```python
from build123d import *

# Parameters (mm, degrees)
SKETCH1_W            = 80
SKETCH1_H            = 50
BOSS_EXTRUDE1_DEPTH  = 90
SKETCH2_W            = 20
SKETCH2_H            = 30
CUT_EXTRUDE1_DEPTH   = 90
BOSS_EXTRUDE2_DEPTH  = 20
CUT_EXTRUDE2_DEPTH   = 127
BOSS_EXTRUDE10_DEPTH = 38
BOSS_EXTRUDE16_DEPTH = 38
BOSS_EXTRUDE17_DEPTH = 38
SKETCH13_W           = 30
SKETCH13_H           = 50
CUT_EXTRUDE4_DEPTH   = 38
SKETCH14_W           = 100
SKETCH14_H           = 90
CUT_EXTRUDE5_DEPTH   = 38
SKETCH15_W           = 106.776830175
SKETCH15_H           = 78.518203409
CUT_EXTRUDE6_DEPTH   = 38
BOSS_EXTRUDE18_DEPTH = 10
CUT_EXTRUDE7_DEPTH   = 10
BOSS_EXTRUDE19_DEPTH = 112
SKETCH19_W           = 80
SKETCH19_H           = 90
CUT_EXTRUDE8_DEPTH   = 112
SKETCH20_W           = 107.666200856
SKETCH20_H           = 176.074092784
CUT_EXTRUDE9_DEPTH   = 112
SKETCH21_W           = 20
SKETCH21_H           = 60
CUT_EXTRUDE10_DEPTH  = 112
SKETCH27_W           = 22.568644797
SKETCH27_H           = 9.839278278
BOSS_EXTRUDE22_DEPTH = 20
BOSS_EXTRUDE24_DEPTH = 91
SKETCH32_W           = 16.460176991
SKETCH32_H           = 60
CUT_EXTRUDE13_DEPTH  = 101
CUT_EXTRUDE14_DEPTH  = 101
BOSS_EXTRUDE25_DEPTH = 5
SKETCH35_W           = 20
SKETCH35_H           = 60
CUT_EXTRUDE15_DEPTH  = 152
BOSS_EXTRUDE27_DEPTH = 20
SKETCH42_W           = 25
SKETCH42_H           = 10
BOSS_EXTRUDE29_DEPTH = 20
BOSS_EXTRUDE30_DEPTH = 20
BOSS_EXTRUDE31_DEPTH = 20
SKETCH46_W           = 60
SKETCH46_H           = 50
CUT_EXTRUDE19_DEPTH  = 20
CUT_EXTRUDE20_DEPTH  = 20
CUT_EXTRUDE21_DEPTH  = 10


with BuildPart() as part:
    # Sketch1 → Boss-Extrude1 (new body)
    with BuildSketch(Plane(origin=(0, 0, 0), x_dir=(1, 0, 0), z_dir=(0, 1, 0))):
        with Locations((40, 25)):
            Rectangle(SKETCH1_W, SKETCH1_H)
    extrude(amount=BOSS_EXTRUDE1_DEPTH)

    # Sketch2 → Cut-Extrude1 (cut)
    with BuildSketch(Plane(origin=(0, 90, 0), x_dir=(1, 0, 0), z_dir=(0, 1, 0))):
        with Locations((10, 15)):
            Rectangle(SKETCH2_W, SKETCH2_H)
    extrude(amount=-CUT_EXTRUDE1_DEPTH, mode=Mode.SUBTRACT)

    # Sketch3 → Boss-Extrude2 (add)
    with BuildSketch(Plane(origin=(80, 0, 0), x_dir=(0, 0, -1), z_dir=(1, 0, 0))):
        Polygon((20, 0), (50, 0), (50, 40), (30, 40), align=None)
    extrude(amount=BOSS_EXTRUDE2_DEPTH)

    # Sketch4 → Cut-Extrude2 (cut)
    with BuildSketch(Plane(origin=(0, 90, 0), x_dir=(1, 0, 0), z_dir=(0, 1, 0))):
        Polygon((60, 0), (80, 20), (80, 0), align=None)
    extrude(amount=-CUT_EXTRUDE2_DEPTH, mode=Mode.SUBTRACT)

    # Sketch7 → Boss-Extrude10 (add)
    with BuildSketch(Plane(origin=(38.787878788, 9.696969697, 38.787878788), x_dir=(0.717740563, -0.168880132, -0.675520529), z_dir=(0.696310624, 0.174077656, 0.696310624))):
        Polygon((29.554023164, -4.850712501), (85.284466846, 4.850712501), (85.284466846, 46.081768757), align=None)
    extrude(amount=-BOSS_EXTRUDE10_DEPTH)

    # Sketch10 → Boss-Extrude16 (add)
    with BuildSketch(Plane(origin=(39.036144578, 8.674698795, 39.036144578), x_dir=(0.715575428, -0.15153362, -0.68190129), z_dir=(0.698535473, 0.155230105, 0.698535473))):
        Polygon((57.246034218, 92.195444573), (15.321732688, 85.687530838), (29.296499865, -4.338609156), (85.195568572, 4.338609156), (85.195568572, 46.23657111), align=None)
    extrude(amount=-BOSS_EXTRUDE16_DEPTH)

    # Sketch11 → Boss-Extrude17 (add)
    with BuildSketch(Plane(origin=(100, 0, 0), x_dir=(0, 0, -1), z_dir=(1, 0, 0))):
        Polygon((20, 0), (29.088944068, 40.900248307), (30, 40), align=None)
    extrude(amount=-BOSS_EXTRUDE17_DEPTH)

    # Sketch13 → Cut-Extrude4 (cut)
    with BuildSketch(Plane(origin=(80, 0, 0), x_dir=(0, 0, -1), z_dir=(1, 0, 0))):
        with Locations((35, 65)):
            Rectangle(SKETCH13_W, SKETCH13_H)
    extrude(amount=CUT_EXTRUDE4_DEPTH, mode=Mode.SUBTRACT)

    # Sketch14 → Cut-Extrude5 (cut)
    with BuildSketch(Plane(origin=(0, 0, -50), x_dir=(-1, 0, 0), z_dir=(0, 0, -1))):
        with Locations((-50, 45)):
            Rectangle(SKETCH14_W, SKETCH14_H)
    extrude(amount=CUT_EXTRUDE5_DEPTH, mode=Mode.SUBTRACT)

    # Sketch15 → Cut-Extrude6 (cut)
    with BuildSketch(Plane.XZ):
        with Locations((53.388415088, -10.740898295)):
            Rectangle(SKETCH15_W, SKETCH15_H)
    extrude(amount=CUT_EXTRUDE6_DEPTH, mode=Mode.SUBTRACT)

    # Sketch16 → Boss-Extrude18 (add)
    with BuildSketch(Plane(origin=(0, 0, 0), x_dir=(-1, 0, 0), z_dir=(0, -1, 0))):
        Polygon((-60, -20), (-60, -40), (-40, -70), (0, -70), (0, -30), (-20, -30), (-20, 0), (-40, 0), align=None)
    extrude(amount=-BOSS_EXTRUDE18_DEPTH)

    # Sketch17 → Cut-Extrude7 (cut)
    with BuildSketch(Plane(origin=(0, 39.026548673, 44.601769912), x_dir=(-1, 0, 0), z_dir=(0, -0.658504608, -0.752576695))):
        Polygon((-20, 67.731902524), (0, -38.569555604), (-40, -38.569555604), (-60, 67.731902524), align=None)
    extrude(amount=-CUT_EXTRUDE7_DEPTH, mode=Mode.SUBTRACT)

    # Sketch18 → Boss-Extrude19 (add)
    with BuildSketch(Plane(origin=(0, 39.026548673, 44.601769912), x_dir=(-1, 0, 0), z_dir=(0, -0.658504608, -0.752576695))):
        Polygon((-20, 67.731902524), (-60, 67.731902524), (-40, -38.569555604), (0, -38.569555604), align=None)
    extrude(amount=BOSS_EXTRUDE19_DEPTH)

    # Sketch19 → Cut-Extrude8 (cut)
    with BuildSketch(Plane(origin=(0, 0, -50), x_dir=(-1, 0, 0), z_dir=(0, 0, -1))):
        with Locations((-40, 45)):
            Rectangle(SKETCH19_W, SKETCH19_H)
    extrude(amount=CUT_EXTRUDE8_DEPTH, mode=Mode.SUBTRACT)

    # Sketch20 → Cut-Extrude9 (cut)
    with BuildSketch(Plane.XZ):
        with Locations((53.833100428, -18.037046392)):
            Rectangle(SKETCH20_W, SKETCH20_H)
    extrude(amount=CUT_EXTRUDE9_DEPTH, mode=Mode.SUBTRACT)

    # Sketch21 → Cut-Extrude10 (cut)
    with BuildSketch(Plane(origin=(0, 0, 0), x_dir=(-1, 0, 0), z_dir=(0, -1, 0))):
        with Locations((-10, 0)):
            Rectangle(SKETCH21_W, SKETCH21_H)
    extrude(amount=-CUT_EXTRUDE10_DEPTH, mode=Mode.SUBTRACT)

    # Sketch27 → Boss-Extrude22 (add)
    with BuildSketch(Plane(origin=(60, 0, 0), x_dir=(0, 0, -1), z_dir=(1, 0, 0))):
        with Locations((-28.715677602, 4.919639139)):
            Rectangle(SKETCH27_W, SKETCH27_H)
    extrude(amount=-BOSS_EXTRUDE22_DEPTH)

    # Sketch31 → Boss-Extrude24 (add)
    with BuildSketch(Plane(origin=(0, 39.026548673, 44.601769912), x_dir=(-1, 0, 0), z_dir=(0, -0.658504608, -0.752576695))):
        Polygon((0, -38.569555604), (-11.428571429, 22.174134755), (0, 22.174134755), align=None)
    extrude(amount=BOSS_EXTRUDE24_DEPTH)

    # Sketch32 → Cut-Extrude13 (cut)
    with BuildSketch(Plane(origin=(0, 0, 0), x_dir=(-1, 0, 0), z_dir=(0, -1, 0))):
        with Locations((-11.769911504, 0)):
            Rectangle(SKETCH32_W, SKETCH32_H)
    extrude(amount=-CUT_EXTRUDE13_DEPTH, mode=Mode.SUBTRACT)

    # Sketch33 → Cut-Extrude14 (cut)
    with BuildSketch(Plane(origin=(7.008547009, -0.992360638, 0.868315559), x_dir=(0.120555065, -0.017069744, -0.992559872), z_dir=(0.982757328, -0.13915148, 0.121757545))):
        Polygon((-0.652056607, -49.430869531), (39.647779316, -2.565835787), (34.800706646, 1.602223376), (-58.135649667, 0), align=None)
    extrude(amount=-CUT_EXTRUDE14_DEPTH, mode=Mode.SUBTRACT)

    # Sketch34 → Boss-Extrude25 (add)
    with BuildSketch(Plane(origin=(0, 0, 0), x_dir=(-1, 0, 0), z_dir=(0, -1, 0))):
        Polygon((0, -58.571428571), (0, -30), (-3.539823009, -30), align=None)
        Polygon((0, 36.93877551), (0, 50), (-40, 50), (-40, -70), (0, -70), (0, -58.571428571), (-3.539823009, -30), (-20, -30), (-20, 30), (-10.973451327, 30), (-11.428571429, 33.673469388), align=None)
        Polygon((0, -30), (0, 30), (-10.973451327, 30), (-20, 30), (-20, -30), (-3.539823009, -30), align=None)
        Polygon((0, 30), (0, 36.93877551), (-11.428571429, 33.673469388), (-10.973451327, 30), align=None)
    extrude(amount=-BOSS_EXTRUDE25_DEPTH)

    # Sketch35 → Cut-Extrude15 (cut)
    with BuildSketch(Plane(origin=(0, 0, 0), x_dir=(-1, 0, 0), z_dir=(0, -1, 0))):
        with Locations((-10, 0)):
            Rectangle(SKETCH35_W, SKETCH35_H)
    extrude(amount=-CUT_EXTRUDE15_DEPTH, mode=Mode.SUBTRACT)

    # Sketch39 → Boss-Extrude27 (add)
    with BuildSketch(Plane(origin=(60, 0, 40), x_dir=(0.554700196, 0, -0.832050294), z_dir=(0.832050294, 0, 0.554700196))):
        Polygon((0, 10), (0, 40), (-36.055512755, 10), align=None)
    extrude(amount=-BOSS_EXTRUDE27_DEPTH)

    # Sketch42 → Boss-Extrude29 (add)
    with BuildSketch(Plane(origin=(60, 0, 0), x_dir=(0, 0, -1), z_dir=(1, 0, 0))):
        with Locations((-27.5, 5)):
            Rectangle(SKETCH42_W, SKETCH42_H)
    extrude(amount=-BOSS_EXTRUDE29_DEPTH)

    # Sketch43 → Boss-Extrude30 (add)
    with BuildSketch(Plane(origin=(60, 0, 0), x_dir=(0, 0, -1), z_dir=(1, 0, 0))):
        Polygon((-40, 10), (-17.777777778, 10), (0, 90), (-40, 40), align=None)
    extrude(amount=-BOSS_EXTRUDE30_DEPTH)

    # Sketch44 → Boss-Extrude31 (add)
    with BuildSketch(Plane(origin=(0, 39.026548673, 44.601769912), x_dir=(1, 0, 0), z_dir=(0, 0.658504608, 0.752576695))):
        Polygon((40, -38.569555604), (60, 67.731902524), (60, 3.762883474), align=None)
    extrude(amount=-BOSS_EXTRUDE31_DEPTH)

    # Sketch46 → Cut-Extrude19 (cut)
    with BuildSketch(Plane(origin=(0, 0, 0), x_dir=(-1, 0, 0), z_dir=(0, -1, 0))):
        with Locations((-30, -45)):
            Rectangle(SKETCH46_W, SKETCH46_H)
    extrude(amount=CUT_EXTRUDE19_DEPTH, mode=Mode.SUBTRACT)

    # Sketch47 → Cut-Extrude20 (cut)
    with BuildSketch(Plane(origin=(0, 0, -20), x_dir=(-1, 0, 0), z_dir=(0, 0, -1))):
        Polygon((-80, 90), (-80, 40), (-91.111111111, 40), align=None)
    extrude(amount=-CUT_EXTRUDE20_DEPTH, mode=Mode.SUBTRACT)

    # Sketch48 → Cut-Extrude21 (cut)
    with BuildSketch(Plane(origin=(60, 0, 40), x_dir=(0.554700196, 0, -0.832050294), z_dir=(0.832050294, 0, 0.554700196))):
        Polygon((0, 0), (0, 64.446209383), (-38.036246254, 32.223104692), (-36.055512755, 0), align=None)
    extrude(amount=CUT_EXTRUDE21_DEPTH, mode=Mode.SUBTRACT)


solid = part.part
```
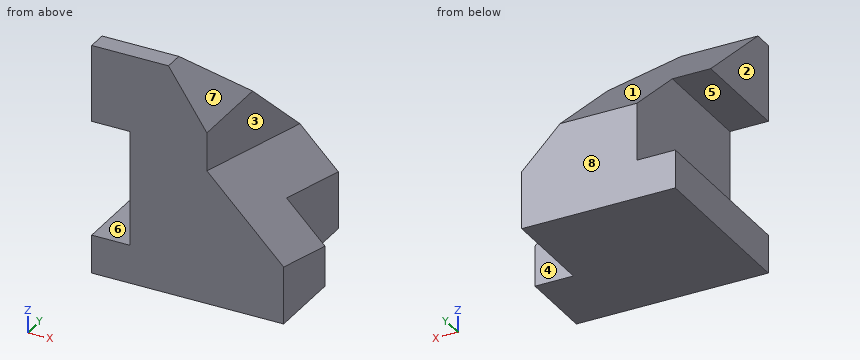
Input: part model. Units: mm. Frame: model coordinates. Face numbers are marked on the shaded views. A direction names the side the tool comes from. Round coordinates to 2 decimals unless told otherwise and drop trailing zeros. Loops run counter-clockwise (first coordinate to the right, second up) from the corner with the lowest first, then second, coordinate; pieces in that order, holes last.
1) Material intervals for line 1 (X direction, y = 59, z = -38.5); line 2 (X direction, y = 34.5, z = 38); line 3 (Z direction, x = 9.5, y = 41) (3 decimals), sorted ascending.
Ans:
line 1: x = 0 to 80
line 2: x = 0 to 60
line 3: z = -50 to -30, 30 to 42.875
2) Set-up query: the marked faces 1, 2, 3, 4 and 5. Return all of +Z, -Z, +X, -X, +Y, -Y with unobstructed straight access to the full face (end or side cutting, diameter ignored); none if empty.
Ans:
face 1: +Z, +X, -X, +Y
face 2: +Z, -Z, -X, +Y, -Y
face 3: +Z, +X, +Y
face 4: +Z, -Z, +X, +Y
face 5: -X, +Y, -Y
3) Section query D-D on x = 53. Return the cut outline in (y, z), plus the area to 3 significant figures.
Ans:
outline: (0, -50) - (90, -50) - (90, 0) - (32.29, 50.5) - (0, 50.5) - close; hole (10, 13) - (31.5, 13) - (10, 17.78) - close
area: 7,540 mm2
4) Pull-direction query (Z, two-part tool) for the marked faces 6, 7 and 8; classes: released by +Z, released by -Z, zero draft, split by the parting line, or undercut.
Ans:
face 6: undercut
face 7: released by +Z
face 8: zero draft
5) Section query A-A on x = 18.5. Return the cut outline in (y, z), plus the area to 3 significant figures.
Ans:
outline: (0, -50) - (90, -50) - (90, -30) - (0, -30) - close; (0, 30) - (55.71, 30) - (10, 70) - (0, 70) - close
area: 3,110 mm2
6) Section query B-B on y = 36. Return the cut outline in (x, z), plus the area to 3 significant figures.
Ans:
outline: (0, -50) - (100, -50) - (100, -28) - (60, 12) - (60, 40) - (55.17, 47.25) - (0, 47.25) - (0, 30) - (20, 30) - (20, -30) - (0, -30) - close; hole (50.87, 12) - (50.99, 10.99) - (52, 12) - close
area: 6,300 mm2
7) Pin query (flat end, axial travel): pin 1 (6 mm diameter, centred on x = 10, y = 43.5, fed in from +Z); pin 2 (10 mm diameter, centred on y = 39.5, z = -20, fed in from -X); pin 3 (1 mm diameter, centred on x = 27, y = 30, fed in from +Z). Return the tip coordinate at first contact, or that it passes through.
Ans:
pin 1: stops at z = 43.31
pin 2: stops at x = 20
pin 3: stops at z = 52.94
8) Section query C-C on z = -38.5. Return the cut outline in (x, y), plus the area to 3 significant figures.
Ans:
outline: (0, 0) - (100, 0) - (100, 40) - (80, 40) - (80, 90) - (0, 90) - close
area: 8,000 mm2
